Source: CAD feature listing. Evaluate the final solid. Frame: model axes, mm. A direction names the side the tool comes from. Round coordinates to 2 decimals unless told otherwise and drop trailing zeros. Loops run counter-clockwise (first coordinate to the right, second up) from the corner with the lowest first, then second, coordinate; pieces in that order, holes last. Notation, with made-up numbers: (54.25, -29) -> (100.25, -29) arc R30 cw to (100.25, -3) -> close; hole circle Ø1 at (84.5, 67.25). An arc over 180 degrees is marked (long way). Return JSON: item names as keys, results as strings. Group by question number.
```python
from build123d import *

# Parameters (mm, degrees)
F1_DEPTH = 1.5


with BuildPart() as f1:
    # F0 (on Front) → F1 (new body, symmetric)
    with BuildSketch(Plane.XZ):
        with BuildLine():
            Line((100, -2.5), (100, 0))
            ThreePointArc((100, 0), (50, 2.187736944), (0, 0))
            ThreePointArc((0, 0), (-13.2819680374, 1.9157530278), (-25.4811713734, 7.5068372317))
            ThreePointArc((-25.4811713734, 7.5068372317), (-13.4145892568, 0.4908203215), (0.2214126109, -2.490177888))
            ThreePointArc((0.2214126109, -2.490177888), (50.0013164202, -0.3122630575), (99.7812101684, -2.4904078382))
            Line((99.7812101684, -2.4904078382), (100, -2.5))
        make_face()
    extrude(amount=F1_DEPTH, both=True)


solid = f1.part
```
(1) Ray query, line 1 (Z direction, x = 47.5, y = -0.75); line 2 (Z direction, x = 65, y = 0.55); line 3 (X direction, y = 1.3, z = 7). Return the intervals inside material, ascending.
(2) Cut plane A-A (y = 0.4). Return loops of the section in (x, z), and give its area (3 significant figures).
(3) Set-up query: faces 1 (the face through (-13.101, -0.021, 1.863)), 2 (the face through (42, 1.5, 0)). Return all of +Z, -Z, +X, -X, +Y, -Y with unobstructed straight access to the full face (end or side cutting, diameter ignored); none if empty.
(4) Mould query, pull axis X, two halves, no side actions, for faces 3 (the face through (42, -1.5, 0)), 4 (the face through (100, 0, -1)), 5 (the face through (50.701, -0.021, 2.187)). Classes: released by +X, released by -X, zero draft, split by the parting line, or undercut.
(5) Cut plane C-C (x = -17). Return loops of the section in (y, z).
Answers follow:
{
 "1": {"line 1": "-0.32 to 2.18", "line 2": "-0.51 to 1.99", "line 3": "-24.85 to -24.68"},
 "2": {"outline": "(-25.48, 7.51) arc R45 ccw to (0.22, -2.49) arc R569.96 cw to (99.78, -2.49) -> (100, -2.5) -> (100, 0) arc R572.46 ccw to (0, 0) arc R47 cw to start", "area": "287 mm^2"},
 "3": {"face 1": "+Z, +Y, -Y", "face 2": "+Z, -Z, +X, -X, +Y"},
 "4": {"face 3": "zero draft", "face 4": "released by +X", "face 5": "undercut"},
 "5": {"outline": "(-1.5, 2.07) -> (1.5, 2.07) -> (1.5, 3.18) -> (-1.5, 3.18) -> close"}
}
